Source: three-view drawing plus pictorial views. Frame: mm from the lowest corner of the part. A direction names the side the tool comes from. Give positions to 0.01 mm unless a question says otherwise; leave off trailing zeros. Write each loop counter-clockwise with the first axis right and the second up, starting at its lowest first coordinate (ties: lowest second). Pieces come first, ordered by that corner, then holes.
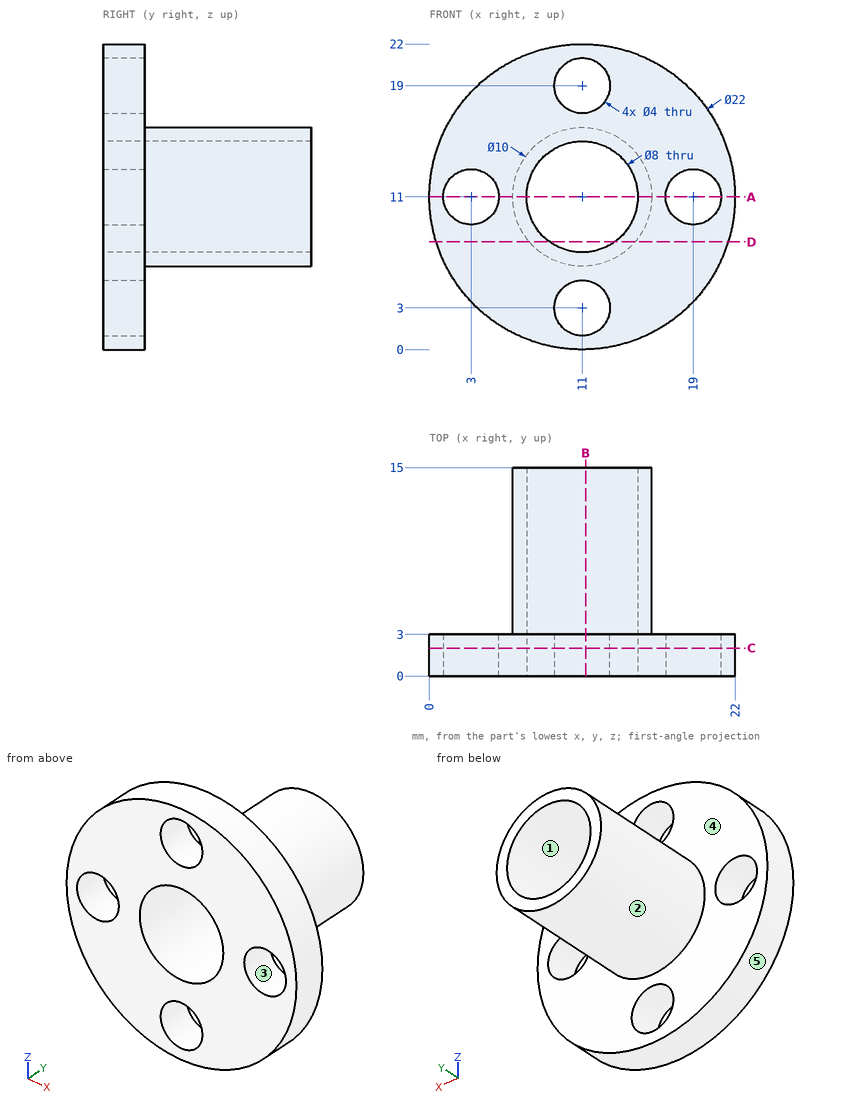
Q1. Section B-B on x = 11.25. Output: boundary loops of the cut face in (y, z), plus the area to 3 significant figures.
Filled sheet:
outline: (0, 0) - (3, 0) - (3, 1.02) - (0, 1.02) - close; (0, 4.98) - (3, 4.98) - (3, 6.01) - (15, 6.01) - (15, 7.01) - (0, 7.01) - close; (0, 14.99) - (15, 14.99) - (15, 15.99) - (3, 15.99) - (3, 17.02) - (0, 17.02) - close; (0, 20.98) - (3, 20.98) - (3, 22) - (0, 22) - close
area: 42.3 mm2
Q2. Pull-direction query (X, two-part tool) for the marked faces 3, 4 and 5; classes: released by +X, released by -X, zero draft, split by the parting line, or undercut.
Filled sheet:
face 3: undercut
face 4: zero draft
face 5: split by the parting line
Q3. Ray query, line 1 along Z through (x, y) = (11, 1.95); line 2 along Y through (x, z) = (7.25, 1.75); line 3 along Z through (x, y) = (8.5, 11.75). Return the intervals inside material, ascending.
Filled sheet:
line 1: z = 0 to 1, 5 to 7, 15 to 17, 21 to 22
line 2: y = 0 to 3
line 3: z = 6.67 to 7.88, 14.12 to 15.33
Q4. Section A-A on z = 11. Output: boundary loops of the cut face in (x, y).
Filled sheet:
outline: (0, 0) - (1, 0) - (1, 3) - (0, 3) - close; (5, 0) - (7, 0) - (7, 15) - (6, 15) - (6, 3) - (5, 3) - close; (15, 0) - (17, 0) - (17, 3) - (16, 3) - (16, 15) - (15, 15) - close; (21, 0) - (22, 0) - (22, 3) - (21, 3) - close
Q5. Section C-C on y = 2. Output: boundary loops of the cut face in (x, z), plus the area to 3 significant figures.
Filled sheet:
outline: circle Ø22 at (11, 11); hole circle Ø4 at (3, 11); hole circle Ø8 at (11, 11); hole circle Ø4 at (11, 3); hole circle Ø4 at (11, 19); hole circle Ø4 at (19, 11)
area: 280 mm2
Q6. Section D-D on z = 7.75. Output: boundary loops of the cut face in (x, y), plus the area to 3 significant figures.
Filled sheet:
outline: (0.49, 0) - (8.67, 0) - (8.67, 15) - (7.2, 15) - (7.2, 3) - (0.49, 3) - close; (13.33, 0) - (21.51, 0) - (21.51, 3) - (14.8, 3) - (14.8, 15) - (13.33, 15) - close
area: 84.3 mm2
Q7. Pin query (flat end, axial travel): P1, Ø5, axis at x = 3, z = 11, coming from the +Y side; P2, Ø10.5, axis at x = 11, z = 11, coming from the +Y side; P3, Ø3.5, axis at x = 11, z = 19, coming from the +Y side; P4, Ø1.5, axis at y = 5, z = 7, coming from the +X side. Return the tip coordinate at first contact, or that it passes through.
Filled sheet:
P1: stops at y = 3
P2: stops at y = 15
P3: passes through
P4: stops at x = 14.8
Q8. Access query for the marked faces 1 and 2. Directions: +Z, -Z, +X, -X, +Y, -Y. A direction counts if a zero-diameter tool reaches every point of the face in a straight line with its end or side. Return the directions, or none.
Filled sheet:
face 1: +Y, -Y
face 2: +Y
